For this review, take the finished solid that the model builds, in its own axes (mm). Coordinates: 2 decimals unless noted, no trailing zeros. Write each loop counter-clockwise with the first axis right and the second up, starting at its lowest first coordinate (ties: lowest second). Pieces come first, ordered by that corner, then holes. Notation, with made-up numbers: (52, 77.25) - (69, 77.25) arc R16 cw to (69, 107.25) - close; hole circle Ø4 at (72, 39). An arc over 180 degrees is marked (long way). Write each question's results on one line, items separated by ' | '.
from build123d import *

# Parameters (mm, degrees)
SKETCH2_W                   = 350
SKETCH2_H                   = 30
BOSS_EXTRUDE1_DEPTH         = 6.35
F_1_4_CLEARANCE_HOLE1_D     = 6.7564
TAP_DRILL_FOR_M3X0_5_TAP1_D = 2.5
LPATTERN1_COUNT             = 6
LPATTERN1_PITCH             = 50


with BuildPart() as part:
    # Sketch2 → Boss-Extrude1 (new body)
    with BuildSketch(Plane.XY):
        with Locations((175, 15)):
            Rectangle(SKETCH2_W, SKETCH2_H)
    extrude(amount=BOSS_EXTRUDE1_DEPTH)

    # 1/4 Clearance Hole1 (through all)
    with Locations(Plane.XY.offset(6.35)):
        with Locations((8, 22), (8, 8)):
            Hole(F_1_4_CLEARANCE_HOLE1_D / 2)

    # Tap Drill for M3x0.5 Tap1 (through all)
    with Locations(Plane.XY.offset(6.35)):
        with Locations((50, 15)):
            tap_drill_for_m3x0_5_tap1 = Hole(TAP_DRILL_FOR_M3X0_5_TAP1_D / 2)

    # LPattern1: Tap Drill for M3x0.5 Tap1 ×6
    with Locations(*[(i * LPATTERN1_PITCH, 0, 0) for i in range(1, LPATTERN1_COUNT)]):
        add(tap_drill_for_m3x0_5_tap1, mode=Mode.SUBTRACT)


solid = part.part
Q1. Wall thickness on line 1 along Y through (x, z) = (250, 4.25); line 2 along X through (y, z) = (21.5, 2.5); line 3 along X through (y, z) = (6.5, 4.5): over which ranges is each line inside the solid? List them lowest first. Write a range as from..to.
Results found:
line 1: 0..13.75, 16.25..30 | line 2: 0..4.66, 11.34..350 | line 3: 0..4.97, 11.03..350
Q2. Take a section at A-A on y = 22. State the section outline as (x, z) points.
Results found:
outline: (0, 0) - (4.62, 0) - (4.62, 6.35) - (0, 6.35) - close; (11.38, 0) - (350, 0) - (350, 6.35) - (11.38, 6.35) - close
Q3. Mouldability with a two-part tool opening along X and no side actions: class faces 1 (the face through (10.49, 10.283, 3.131)), 2 (the face through (8.44, 25.35, 3.13)), 3 (the face through (350, 15, 3)), 4 (the face through (173, 30, 3)) as pulls with the +X half, pulls with the -X half, needs draft (parallel to the pull), parting line crosses it, or undercut.
Results found:
face 1: undercut | face 2: undercut | face 3: pulls with the +X half | face 4: needs draft
